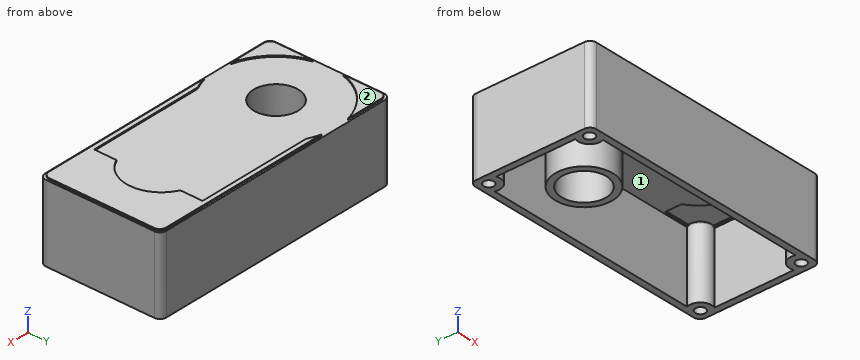
```python
from build123d import *

# Parameters (mm, degrees)
CROQUIS1_R              = 3.5
CROQUIS1_R_2            = 0.8
SALIENTE_EXTRUIR1_DEPTH = 12
SALIENTE_EXTRUIR2_DEPTH = 0.2
VACIADO6_OUTLINE_R      = 4.5
VACIADO6_DEPTH          = 11
VACIADO6_START          = 11
VACIADO6_2_DEPTH        = 0.2


# Read off the part's stored shape, not the designer's step: Vaciado6
with BuildPart() as part:
    # Croquis1 → Saliente-Extruir1 (new body)
    with BuildSketch(Plane.XY):
        with BuildLine():
            Line((-9.5, 8.5), (-9.5, -8.5))
            ThreePointArc((-9.5, -8.5), (-9.207106781, -9.207106781), (-8.5, -9.5))
            Line((-8.5, -9.5), (30, -9.5))
            ThreePointArc((30, -9.5), (30.707106781, -9.207106781), (31, -8.5))
            Line((31, -8.5), (31, 8.5))
            ThreePointArc((31, 8.5), (30.707106781, 9.207106781), (30, 9.5))
            Line((30, 9.5), (-8.5, 9.5))
            ThreePointArc((-8.5, 9.5), (-9.207106781, 9.207106781), (-9.5, 8.5))
        make_face()
        Circle(CROQUIS1_R, mode=Mode.SUBTRACT)
        with Locations((29.4, -7.9)):
            Circle(CROQUIS1_R_2, mode=Mode.SUBTRACT)
        with Locations((-7.9, -7.9)):
            Circle(CROQUIS1_R_2, mode=Mode.SUBTRACT)
        with Locations((-7.9, 7.9)):
            Circle(CROQUIS1_R_2, mode=Mode.SUBTRACT)
        with Locations((29.4, 7.9)):
            Circle(CROQUIS1_R_2, mode=Mode.SUBTRACT)
    extrude(amount=SALIENTE_EXTRUIR1_DEPTH)

    # Croquis2 → Saliente-Extruir2 (add)
    with BuildSketch(Plane.XY.offset(12)):
        with BuildLine():
            Line((2.368543856, -9.2), (29.7, -9.2))
            ThreePointArc((29.7, -9.2), (30.407106781, -8.907106781), (30.7, -8.2))
            Line((30.7, -8.2), (30.7, 8.2))
            ThreePointArc((30.7, 8.2), (30.407106781, 8.907106781), (29.7, 9.2))
            Line((29.7, 9.2), (2.368543856, 9.2))
            ThreePointArc((2.368543856, 9.2), (3.324069835, 8.899469632), (4.242640687, 8.5))
            Line((4.242640687, 8.5), (22.5, 8.5))
            Line((22.5, 8.5), (22.5, 5))
            ThreePointArc((22.5, 5), (25.7, 0), (22.5, -5))
            Line((22.5, -5), (22.5, -8.5))
            Line((22.5, -8.5), (4.242640687, -8.5))
            ThreePointArc((4.242640687, -8.5), (3.324069835, -8.899469632), (2.368543856, -9.2))
        make_face()
        with BuildLine():
            Line((-8.2, -9.2), (-2.368543856, -9.2))
            ThreePointArc((-2.368543856, -9.2), (-6.717514421, -6.717514421), (-9.2, -2.368543856))
            Line((-9.2, -2.368543856), (-9.2, -8.2))
            ThreePointArc((-9.2, -8.2), (-8.907106781, -8.907106781), (-8.2, -9.2))
        make_face()
        with BuildLine():
            Line((-9.2, 8.2), (-9.2, 2.368543856))
            ThreePointArc((-9.2, 2.368543856), (-6.717514421, 6.717514421), (-2.368543856, 9.2))
            Line((-2.368543856, 9.2), (-8.2, 9.2))
            ThreePointArc((-8.2, 9.2), (-8.907106781, 8.907106781), (-9.2, 8.2))
        make_face()
    extrude(amount=SALIENTE_EXTRUIR2_DEPTH)

    # Vaciado6 outline → Vaciado6 (cut)
    with BuildSketch(Plane.XY):
        with BuildLine():
            Line((27.702943725, 8.5), (-6.202943725, 8.5))
            ThreePointArc((-6.202943725, 8.5), (-6.627207794, 6.627207794), (-8.5, 6.202943725))
            Line((-8.5, 6.202943725), (-8.5, -6.202943725))
            ThreePointArc((-8.5, -6.202943725), (-6.627207794, -6.627207794), (-6.202943725, -8.5))
            Line((-6.202943725, -8.5), (27.702943725, -8.5))
            ThreePointArc((27.702943725, -8.5), (28.127207794, -6.627207794), (30, -6.202943725))
            Line((30, -6.202943725), (30, 6.202943725))
            ThreePointArc((30, 6.202943725), (28.127207794, 6.627207794), (27.702943725, 8.5))
        make_face()
        Circle(VACIADO6_OUTLINE_R, mode=Mode.SUBTRACT)
    extrude(amount=VACIADO6_DEPTH, mode=Mode.SUBTRACT)

    # Vaciado6 2 outline → Vaciado6 2 (cut)
    with BuildSketch(Plane.XY.offset(VACIADO6_START)):
        with BuildLine():
            ThreePointArc((29.7, 6.125176065), (28.127207794, 6.627207794), (27.625176065, 8.2))
            Line((27.625176065, 8.2), (23.5, 8.2))
            Line((23.5, 8.2), (23.5, 5.60357029))
            ThreePointArc((23.5, 5.60357029), (26.7, 0), (23.5, -5.60357029))
            Line((23.5, -5.60357029), (23.5, -8.2))
            Line((23.5, -8.2), (27.625176065, -8.2))
            ThreePointArc((27.625176065, -8.2), (28.127207794, -6.627207794), (29.7, -6.125176065))
            Line((29.7, -6.125176065), (29.7, 6.125176065))
        make_face()
    extrude(amount=VACIADO6_2_DEPTH, mode=Mode.SUBTRACT)


solid = part.part
```
Could you check a few things on this model? Use its own coordinates, in mm. Face numbers are marked on the shaded views. A direction names the side the tool comes from. Round coordinates to 2 decimals unless told otherwise and drop trailing zeros. Write each loop counter-clockwise with the first axis right and the second up, starting at its lowest first coordinate (ties: lowest second). Pieces come first, ordered by that corner, then holes. Notation, with made-up numbers: M 4,55.5 L 36,55.5 A13 ccw 36,62.5 Z; hole C -10.75,24 d2. An arc over 180 degrees is marked long. Write each question's results on one line, items separated by ' | '. Start each with the question number.
1. I'm going to push flat-ended pins straight in: pin 1 Ø0.5 at (x, y) = (29.5, 7.5) entering from -Z; pin 2 Ø6 at (x, y) = (17, 0.5) entering from +Z; pin 3 Ø1 at (x, y) = (24.5, 6.5) entering from -Z. Where does each tip first touch, or does it pass through?
2. Imagine slicing it at B-B on z = 3.25. List the corners of the cut face in (x, y) for me, and give its area (3 significant figures).
3. Imagine slicing it at D-D on x = 18. List the corners of the cut face in (y, z) for me.
4. Imagine slicing it at C-C on y = 0. List the corners of the cut face in (x, z) for me, and give its area (3 significant figures).
5. I need wall thicknesses on L1, parallel to Y at x = 29.4, z = 5; L2, parallel to X at y = -8, z = 6; L3, parallel to X at y = 4, z = 1.25. Which ranges of each line are inside material? Lowest first, please. Write a range as from..to.
6. On a 3-axis mill with a long thin cutter (end or side, diameter ignored), from which of +Z, -Z, +X, -X, +Y, -Y can I reach the whole of each face in a straight line? I mean the marked faces 1 and 2. Say none if no direction works.
7. Imagine slicing it at A-A on x = 0. List the corners of the cut face in (y, z) for me, and give its area (3 significant figures).
Result sheet:
1) pin 1: stops at z = 12 | pin 2: stops at z = 12 | pin 3: stops at z = 11.2
2) outline: M -9.5,-8.5 A1 ccw -8.5,-9.5 L 30,-9.5 A1 ccw 31,-8.5 L 31,8.5 A1 ccw 30,9.5 L -8.5,9.5 A1 ccw -9.5,8.5 Z; C 0,0 d9; hole C -7.9,-7.9 d1.6; hole C -7.9,7.9 d1.6; hole M -8.5,-6.2 A1.8 cw -6.2,-8.5 L 27.7,-8.5 A1.8 cw 30,-6.2 L 30,6.2 A1.8 cw 27.7,8.5 L -6.2,8.5 A1.8 cw -8.5,6.2 Z; hole C 0,0 d7; hole C 29.4,-7.9 d1.6; hole C 29.4,7.9 d1.6 | area: 151 mm^2
3) outline: M -9.5,0 L -8.5,0 L -8.5,11 L 8.5,11 L 8.5,0 L 9.5,0 L 9.5,12 L 9.2,12 L 9.2,12.2 L 8.5,12.2 L 8.5,12 L -8.5,12 L -8.5,12.2 L -9.2,12.2 L -9.2,12 L -9.5,12 Z
4) outline: M -9.5,0 L -8.5,0 L -8.5,11 L -4.5,11 L -4.5,0 L -3.5,0 L -3.5,12 L -9.5,12 Z; M 3.5,0 L 4.5,0 L 4.5,11 L 26.7,11 L 26.7,11.2 L 29.7,11.2 L 29.7,11 L 30,11 L 30,0 L 31,0 L 31,12 L 30.7,12 L 30.7,12.2 L 25.7,12.2 L 25.7,12 L 3.5,12 Z | area: 77.9 mm^2
5) L1: y = -9.5..-8.7, -7.1..-6.1, 6.1..7.1, 8.7..9.5 | L2: x = -9.5..-8.69, -7.11..-6.1, 27.6..28.61, 30.19..31 | L3: x = -9.5..-8.5, -2.06..2.06, 30..31
6) face 1: -Z | face 2: +Z, +X, -X, +Y, -Y
7) outline: M -9.5,0 L -8.5,0 L -8.5,11 L -4.5,11 L -4.5,0 L -3.5,0 L -3.5,12 L -9.5,12 Z; M 3.5,0 L 4.5,0 L 4.5,11 L 8.5,11 L 8.5,0 L 9.5,0 L 9.5,12 L 3.5,12 Z | area: 56.0 mm^2
